Check sheet for the modelled part. Datum: model origin and axes. Units: mm. Face numbers are marked on the shaded views. A direction names the side the tool comes from. Coordinates: 2 decimals unless noted, no trailing zeros. Loops run counter-clockwise (first coordinate to the right, second up) from the corner with the lowest first, then second, coordinate; pieces in that order, holes last. Notation, with made-up numbers: (43, 60.25) -> (84, 60.25) arc R23 ccw to (84, 80.25) -> close; hole circle Ø1 at (18.25, -18). An arc over 180 degrees is marked (long way). Use CSV: the item, a comma, the result in double quotes.
Autodesk Inventor part; units mm, degrees
ref_plane "YZ Plane" through (0, 0, 0) normal (1, 0, 0) x (0, 1, 0)
ref_plane "XZ Plane" through (0, 0, 0) normal (0, 1, 0) x (-1, 0, 0)
ref_plane "XY Plane" through (0, 0, 0) normal (0, 0, 1) x (1, 0, 0)
sketch "Sketch1" plane through (0, 0, 0) normal (0, 0, 1) x (1, 0, 0)
  line L0 (0, 0) -> (45, 0)
  line L1 (45, 0) -> (45, -95)
  line L2 (45, -95) -> (0, -95)
  line L3 (0, -95) -> (0, 0)
  dimension "d14" = 95
  dimension "d15" = 45
extrude "Extrusion1" add sketch "Sketch1" against normal blind 30
sketch "Sketch2" plane through (0, 0, -30) normal (0, 0, -1) x (-1, 0, 0)
  line L0 (0, -95) -> (0, 0)
  line L1 (0, 0) -> (-12, 0)
  line L2 (-12, 0) -> (-12, -95)
  line L3 (-12, -95) -> (0, -95)
  line L4 (0, -95) -> (0, 0)
  line L5 (-45, -95) -> (0, -95)
  dimension "d2" = 12
extrude "Extrusion2" cut sketch "Sketch2" against normal blind 20
sketch "Sketch3" plane through (45, -95, 0) normal (1, 0, 0) x (0, 0, -1)
  circle A0 centre (25.875, 47.5) radius 15.621 construction
  circle A1 centre (25.875, 47.5) radius 12.5
  line L0 (0, 0) -> (0, 95) construction
  line L1 (0, 0) -> (30, 0)
  line L2 (30, 0) -> (0, 95) construction
  line L3 (30, 95) -> (0, 0) construction
  point P0 (15, 47.5)
  point P1 (10, 95)
  dimension "d5" = 31.242
  dimension "d6" = 25
  dimension "d13" = 15.875
extrude "Extrusion3" cut sketch "Sketch3" against normal through all
sketch "Sketch4" plane through (12, 0, -10) normal (-1, 0, 0) x (0, 0, 1)
  arc A0 (-20, -59.2998) -> (-20, -35.7002) centre (-15.875, -47.5) ccw
  circle A1 centre (-15.875, -47.5) radius 20
  point P0 (10, 0)
  dimension "d9" = 40
extrude "Extrusion4" cut sketch "Sketch4" against normal blind 13
sketch "Sketch5" plane through (45, -95, 0) normal (1, 0, 0) x (0, 0, -1)
  arc A0 (15, 84.9933) -> (22.5, 77.4933) centre (22.5, 84.9933) ccw
  circle A1 centre (22.5, 84.9933) radius 2.5 construction
  line L0 (22.5, 77.4933) -> (30, 77.4933)
  line L1 (30, 95) -> (30, 59.2998)
  line L2 (15, 84.9933) -> (15, 95)
  line L3 (0, 95) -> (30, 95)
  point P0 (15.0002, 95)
  dimension "d17" = 15
extrude "Extrusion5" cut sketch "Sketch5" against normal blind 25
sketch "Sketch6" plane through (20, -95, 0) normal (1, 0, 0) x (0, 0, -1)
  arc A0 (15, 84.9933) -> (22.5, 77.4933) centre (22.5, 84.9933) ccw
  circle A1 centre (22.5, 84.9933) radius 3
  point P0 (0, 95)
  point P1 (15.0002, 95)
  dimension "d20" = 6
extrude "Extrusion6" cut sketch "Sketch6" against normal through all
ref_plane "Work Plane1" through (0, -47.5, 0) normal (0, 1, 0) x (1, 0, 0)
mirror "Mirror1" about plane through (0, -47.5, 0) normal (0, 1, 0) of "Extrusion5", "Extrusion6"
chamfer "Chamfer3" distance 6 angle 45 2 edges at (35, -59.2998, -30) (35, -35.7002, -30)
chamfer "Chamfer1" distance 2 angle 45 20 edges at (45, -5.0033, -15) (45, -15.31, -17.1967) (45, -17.5067, -26.25) (45, -89.9967, -15) (45, -79.69, -17.1967) (45, -77.4933, -26.25) (16, 0, -30) (16, -95, -30) (45, 0, -7.5) (6, 0, -10) (45, -95, -7.5) (6, -95, -10) (45, -23.6034, -30) (45, -47.5, -13.375) (45, -71.3966, -30) (25, -47.5, -13.375) (12, -28.7443, -18.9306) (12, -66.2557, -18.9306) (45, -32.4188, -27.0132) (45, -62.5812, -27.0132)
chamfer "Chamfer2" distance 1 angle 45 2 edges at (20, -10.0067, -19.5) (20, -84.9933, -19.5)
properties part number "pillar_placer"
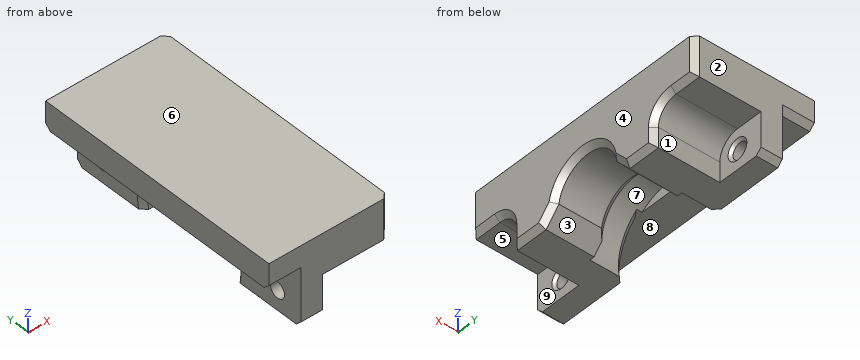
1) Draft check along Z on the marked faces 6, 7, 8 and 9. Enter one of: released by +Z, released by -Z, zero draft, split by the parting line, or undercut.
Answer below:
face 6,"released by +Z"
face 7,"undercut"
face 8,"released by -Z"
face 9,"zero draft"
2) Thickness scan on line 1 along Y through (x, z) = (16, -22); line 2 along Z through (x, y) = (17.25, -47.5) (3 decimals); line 3 along X through (y, z) = (-31, -16). Record the ranges inside material, lowest first. Write a range as from..to.
Answer below:
line 1,"y = -95..-87.95, -82.04..-67.12, -27.88..-12.96, -7.05..0"
line 2,"z = -5.875..0"
line 3,"x = 25..45"
3) Cross-section at C-C on x = 34. Record the boundary of the cut face in (y, z) (3 decimals).
Answer below:
outline,"(-95, -15) -> (-84.993, -15) arc R7.5 cw to (-77.493, -22.5) -> (-77.493, -30) -> (-65.3, -30) -> (-59.863, -24.026) arc R12.5 cw to (-35.137, -24.026) -> (-29.7, -30) -> (-17.507, -30) -> (-17.507, -22.5) arc R7.5 cw to (-10.007, -15) -> (0, -15) -> (0, 0) -> (-95, 0) -> close"
4) Cross-section at D-D on x = 16. Record the boundary of the cut face in (y, z) (3 decimals), and give its area (3 significant figures).
Answer below:
outline,"(-95, -28) -> (-93, -30) -> (-67.07, -30) arc R20 cw (long way) to (-27.93, -30) -> (-2, -30) -> (0, -28) -> (0, 0) -> (-95, 0) -> close; hole circle Ø6 at (-84.993, -22.5); hole circle Ø6 at (-10.007, -22.5)"
area,"2,000 mm²"
5) Go/stop test with flat-tipped pins: pin 1 Ø7.5 at (y, z) = (-12.5, -26) entering from +X; pin 2 Ø8 at (x, z) = (30.5, -25.5) entering from -Y; pin 3 Ø11 at (x, y) = (35.5, -92) entering from -Z; pin 4 Ø5 at (y, z) = (-84.99, -22.5) entering from +X. Record where each tip stops, or that it passes through.
Answer below:
pin 1,"stops at x = 20"
pin 2,"stops at y = -77.56"
pin 3,"stops at z = -15"
pin 4,"passes through"
6) Cross-section at A-A on z = -7. Record the boundary of the cut face in (x, y).
Answer below:
outline,"(0, -95) -> (43, -95) -> (45, -93) -> (45, -2) -> (43, 0) -> (0, 0) -> close; hole (12, -54.11) -> (25, -54.11) -> (25, -40.89) -> (12, -40.89) -> close"
7) Access from +Z, -Z, +X, -X, +Y, -Y to the whole of each face (thin tool, end or side, straight path). Record for the marked faces 1, 2, 3, 4 and 5.
Answer below:
face 1,"-Z, +X, +Y"
face 2,"+Z, -Z, +X, -X, +Y"
face 3,"-Z, +X, -X"
face 4,"+Z, -Z, +X, +Y, -Y"
face 5,"-Z, +X, -Y"
8) Cross-section at B-B on y = -47.5. Record the boundary of the cut face in (x, z) (3 decimals), and give its area (3 significant figures).
Answer below:
outline,"(0, -10) -> (12, -10) -> (12, -5.875) -> (25, -5.875) -> (25, -11.375) -> (27, -13.375) -> (43, -13.375) -> (45, -11.375) -> (45, 0) -> (0, 0) -> close"
area,"460 mm²"
